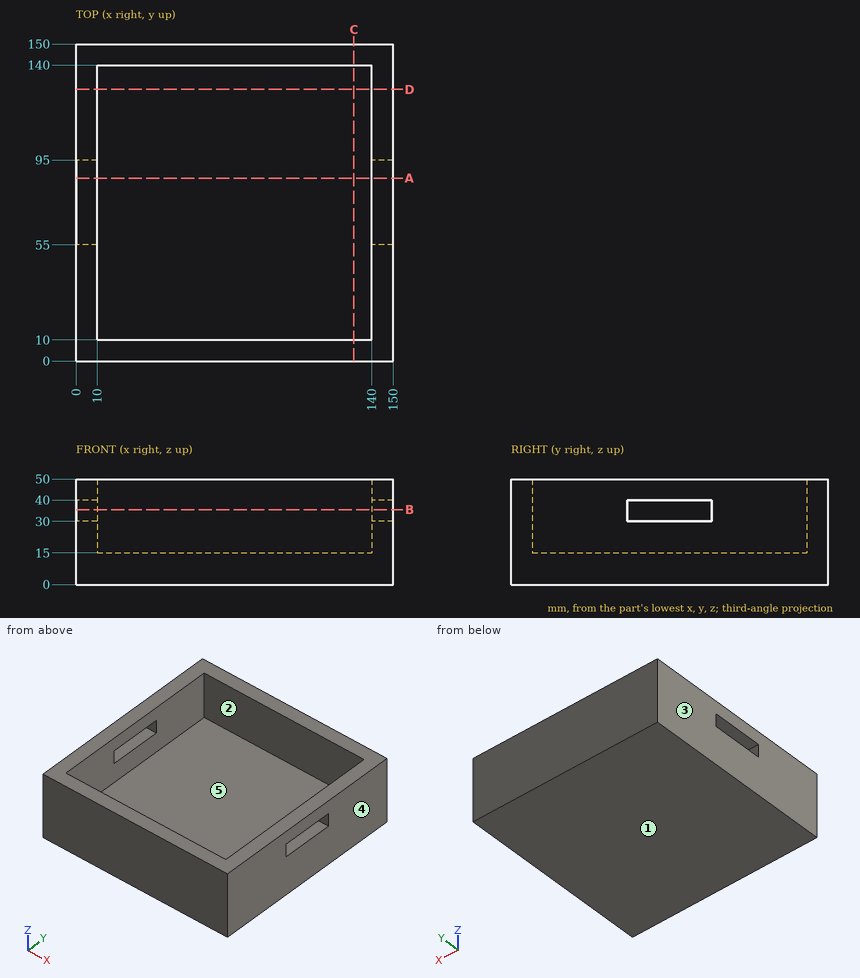
Source: three-view drawing plus pictorial views. Frame: mm from the lowest corner of the part. A direction names the side the tool comes from. Round coordinates to 2 decimals unless told otherwise and drop trailing zeros. Order: outer loops, then holes, each group sorted by start corner. A loop starts at its lowest first (then second) coordinate and runs counter-clockwise, first axis right, second up. Notation, with made-up numbers: (-9.5, -38) -> (37.5, -38) arc R20 ccw to (37.5, -3) -> close; hole circle Ø5 at (-37, 70.25). An arc over 180 degrees is marked (long way). Use one line per item in the form item = value. Start each with the question number.
1. Cut plane B-B (z = 35.5). Return the cut outline in (x, y).
2. Cut plane A-A (y = 86.5). Return the cut outline in (x, z).
3. Pin query (flat end, axial travel): pin 1 Ø3 at (x, y) = (66, 107) entering from +Z. Return the tip coordinate at first contact, or that it passes through.
4. Reachability of the marked faces 4 and 5 from +Z, -Z, +X, -X, +Y, -Y: full face, straight path, thin tool, end or side. Return the list, or none.
5. Draft query along X for the marked faces 1, 2 and 3. Return one class per face: pulls with the +X half, pulls with the -X half, needs draft (parallel to the pull), parting line crosses it, or undercut.
6. Line query: probe 1 along X at (y, z) = (23.5, 37); probe 2 along Y at (x, z) = (8.5, 37). Output: solid intervals per line, ascending.
7. Cut plane C-C (x = 131.5). Return the cut outline in (y, z), then the cut area to 3 significant figures.
Solution:
q1.outline = (0, 0) -> (150, 0) -> (150, 55) -> (140, 55) -> (140, 10) -> (10, 10) -> (10, 55) -> (0, 55) -> close; (0, 95) -> (10, 95) -> (10, 140) -> (140, 140) -> (140, 95) -> (150, 95) -> (150, 150) -> (0, 150) -> close
q2.outline = (0, 0) -> (150, 0) -> (150, 30) -> (140, 30) -> (140, 15) -> (10, 15) -> (10, 30) -> (0, 30) -> close; (0, 40) -> (10, 40) -> (10, 50) -> (0, 50) -> close; (140, 40) -> (150, 40) -> (150, 50) -> (140, 50) -> close
q3.pin_1 = 15
q4.face_4 = +Z, -Z, +X, +Y, -Y
q4.face_5 = +Z
q5.face_1 = needs draft
q5.face_2 = undercut
q5.face_3 = pulls with the -X half
q6.probe_1 = 0 to 10, 140 to 150
q6.probe_2 = 0 to 55, 95 to 150
q7.outline = (0, 0) -> (150, 0) -> (150, 50) -> (140, 50) -> (140, 15) -> (10, 15) -> (10, 50) -> (0, 50) -> close
q7.area = 2,950 mm^2
